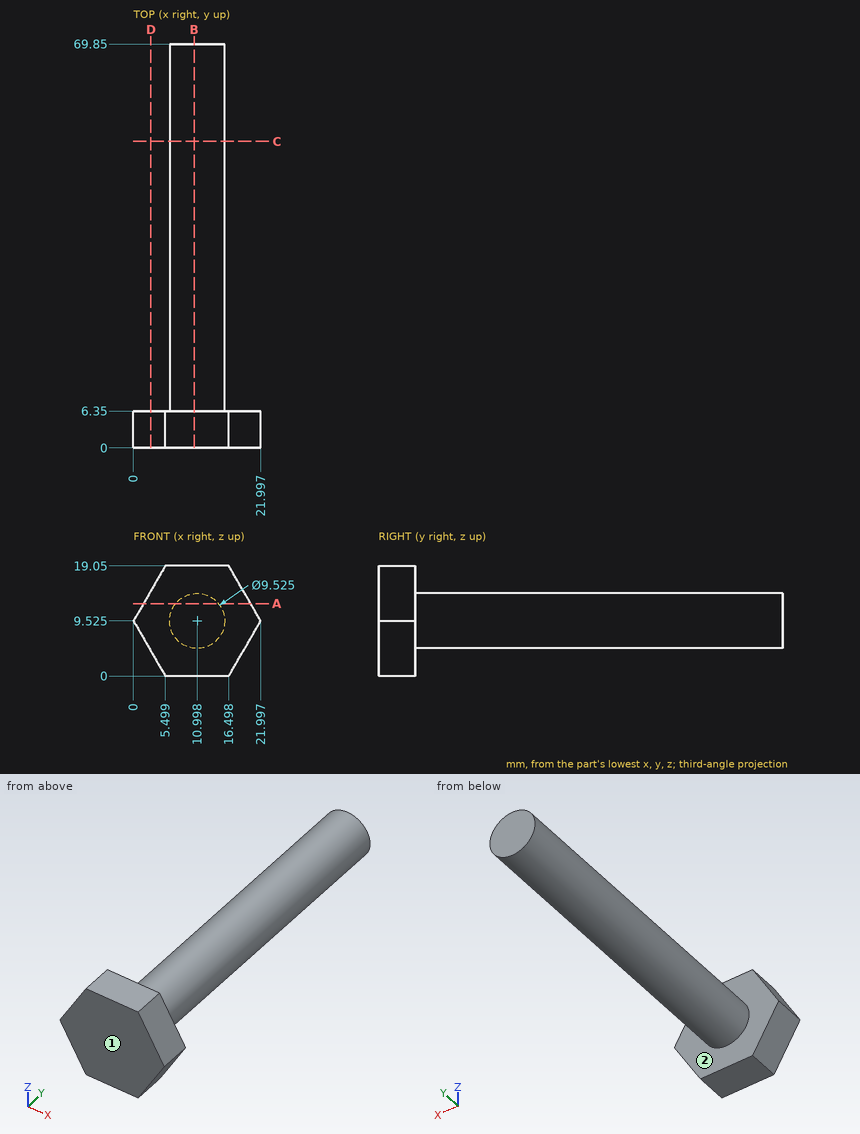
Part print with two shaded views. Sizes in mm from the minimum x, y, z corner. A direction names the side the tool comes from. Round coordinates to 2 decimals unless told otherwise and drop trailing zeros. Order: outer loops, then holes, each group sorted by start corner. A loop starts at its lowest first (then second) coordinate and runs counter-clockwise, first axis right, second up. Notation, with made-up numbers: (73.5, 34.5) - (108.5, 34.5) arc R25 cw to (108.5, 47.5) - close; hole circle Ø2 at (-32, 64). An arc over 180 degrees is marked (long way). Answer as CSV lines item,"result". Start each with the question number.
1. Saw through at D-D, the plane x = 3. Write the cut outline in (y, z).
2. Saw through at A-A, the plane z = 12.5. Write the cut outline in (x, y), and give its area (3 significant figures).
3. Drill centre lines: L1, parallel to Y at x = 16, z = 11.75; L2, parallel to Z at x = 11.25, y = 43; L3, parallel to Z at x = 14.75, y = 66. Where is each one in solid material? Low to high. Write a range as [from, to].
4. Saw through at C-C, the plane y = 53. Write the cut outline in (x, z) (1 decimal).
5. Saw through at B-B, the plane x = 10.5. Write the cut outline in (y, z).
6. Pin check, flat tips, straight feed: pin 1 (6 mm diameter, centred on x = 7, z = 16.5, fed in from +Y); pin 2 (10 mm diameter, centred on x = 19, y = 60, fed in from -Z); pin 3 (4 mm diameter, centred on y = 53, z = 15, fed in from +X) (1 decimal); pin 4 (5 mm diameter, centred on x = 2.5, y = 40, fed in from -Z). Stop position of each tip, or through.
7. Tool access for the marked faces 1 and 2: list every direction of +Z, -Z, +X, -X, +Y, -Y with a clear straight run to the whole face (end or side of a thin tool).
Model answer:
1,outline,"(0, 4.33) - (6.35, 4.33) - (6.35, 14.72) - (0, 14.72) - close"
2,outline,"(1.72, 0) - (20.28, 0) - (20.28, 6.35) - (14.72, 6.35) - (14.72, 69.85) - (7.28, 69.85) - (7.28, 6.35) - (1.72, 6.35) - close"
2,area,"590 mm²"
3,L1,"y = [0, 6.35]"
3,L2,"z = [4.77, 14.28]"
3,L3,"z = [6.59, 12.46]"
4,outline,"circle Ø9.5 at (11, 9.5)"
5,outline,"(0, 0) - (6.35, 0) - (6.35, 4.79) - (69.85, 4.79) - (69.85, 14.26) - (6.35, 14.26) - (6.35, 19.05) - (0, 19.05) - close"
6,pin 1,"stops at y = 6.35"
6,pin 2,"stops at z = 5.83"
6,pin 3,"stops at x = 14.3"
6,pin 4,"passes through"
7,face 1,"+Z, -Z, +X, -X, -Y"
7,face 2,"+Y"
